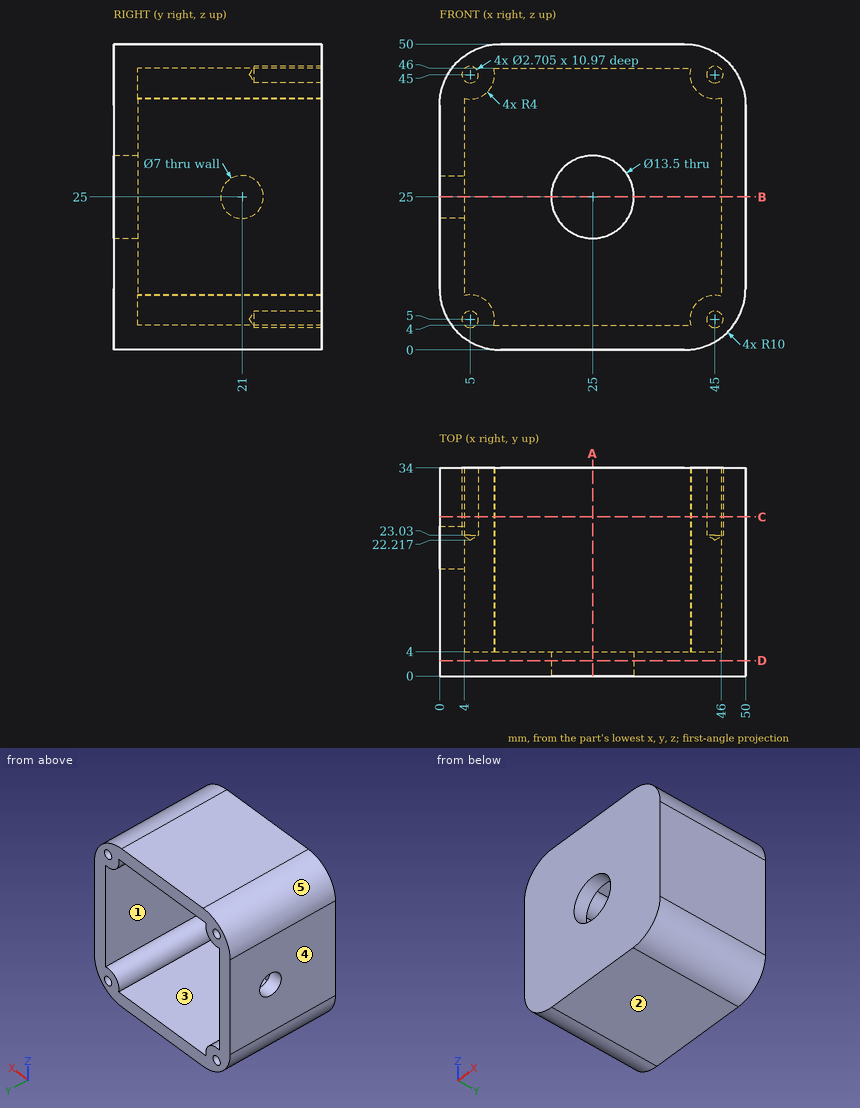
The figure shows three views and two pictorial views of one solid part (mm, origin at its lowest corner). Answer the questions. A direction names the side the tool comes from. Give positions to 0.01 mm unless a question says otherwise; leave off trailing zeros. Order: outer loops, then holes, each group sorted by start corner. A loop starts at its lowest first (then second) coordinate and runs counter-clockwise, first axis right, second up. Notation, with made-up numbers: M 50,-8.75 L 60,-8.75 A31 ccw 60,30.25 Z; hole C -18.75,-39.75 d11. An arc over 180 degrees is marked long. Return JSON: item names as keys, results as strings.
Q1. The mould has two halves that part along Z. Classify the marked faces 3, 4 and 5: pulls with the +Z half, pulls with the -Z half, needs draft (parallel to the pull), parting line crosses it, or undercut.
Answer below:
{"face 3": "undercut", "face 4": "needs draft", "face 5": "pulls with the +Z half"}
Q2. Which of the six approach directions +Z, -Z, +X, -X, +Y, -Y give full straight-line access (tool end or side, diameter ignored) to the marked faces 1 and 2?
Answer below:
{"face 1": "+Y", "face 2": "-Z, +X, -X, +Y, -Y"}
Q3. Find section B-B, the plane z = 25. Write down the section's boundary in (x, y), and give its area (3 significant figures).
Answer below:
{"outline": "M 0,0 L 18.25,0 L 18.25,4 L 4,4 L 4,17.5 L 0,17.5 Z; M 0,24.5 L 4,24.5 L 4,34 L 0,34 Z; M 31.75,0 L 50,0 L 50,34 L 46,34 L 46,4 L 31.75,4 Z", "area": "358 mm^2"}
Q4. Find the intervals of material crossed by line 1 along Y through (x, z) = (1, 25); line 2 along X through (y, z) = (31, 45); line 3 along X through (y, z) = (18, 39.5), in increasing order. Write a range as [from, to].
Answer below:
{"line 1": "y = [0, 17.5], [24.5, 34]", "line 2": "x = [1.34, 3.65], [6.35, 9], [41, 43.65], [46.35, 48.66]", "line 3": "x = [0, 4], [46, 50]"}
Q5. Each of these flat-tipped pins is pushed along its axis until it touches: pin 1 (1 mm diameter, centred on x = 15.5, z = 43.5, fed in from +Y); pin 2 (1 mm diameter, centred on x = 6.5, y = 18.5, fed in from +Z); pin 3 (8 mm diameter, centred on x = 23, z = 24, fed in from +Y). Where does it stop, or does it pass through?
Answer below:
{"pin 1": "stops at y = 4", "pin 2": "stops at z = 49.54", "pin 3": "passes through"}
Q6. Find section D-D, the plane y = 2.5. Write down the section's boundary in (x, z).
Answer below:
{"outline": "M 0,10 A10 ccw 10,0 L 40,0 A10 ccw 50,10 L 50,40 A10 ccw 40,50 L 10,50 A10 ccw 0,40 Z; hole C 25,25 d13.5"}
Q7. Find section A-A, the plane x = 25. Write down the section's boundary in (y, z), and give its area (3 significant figures).
Answer below:
{"outline": "M 0,0 L 34,0 L 34,4 L 4,4 L 4,18.25 L 0,18.25 Z; M 0,31.75 L 4,31.75 L 4,46 L 34,46 L 34,50 L 0,50 Z", "area": "386 mm^2"}
Q8. Find section C-C, the plane y = 26. Write down the section's boundary in (x, z) (1 decimal), and give its area (3 significant figures).
Answer below:
{"outline": "M 0,10 A10 ccw 10,0 L 40,0 A10 ccw 50,10 L 50,40 A10 ccw 40,50 L 10,50 A10 ccw 0,40 Z; hole C 5,5 d2.7; hole C 5,45 d2.7; hole M 4,8.9 A4 cw 8.9,4 L 41.1,4 A4 cw 46,8.9 L 46,41.1 A4 cw 41.1,46 L 8.9,46 A4 cw 4,41.1 Z; hole C 45,5 d2.7; hole C 45,45 d2.7", "area": "713 mm^2"}
